from build123d import *

# Parameters (mm, degrees)
SKETCH1_R               = 3
BOSS_EXTRUDE1_DEPTH     = 33
SKETCH2_W               = 1.5
SKETCH2_H               = 4
FILLET2_R               = 0.5
CUT_EXTRUDE2_DEPTH      = 34.271609528
CUT_EXTRUDE2_DEPTH_BACK = 34.271609528
SKETCH3_R               = 1


with BuildPart() as part:
    # Sketch1 → Boss-Extrude1 (new body)
    with BuildSketch(Plane.XY):
        Circle(SKETCH1_R)
    extrude(amount=BOSS_EXTRUDE1_DEPTH)

    # Sketch2 → Cut-Revolve1 (revolve, cut)
    with BuildSketch(Plane(origin=(0, 0, 0), x_dir=(1, 0, 0), z_dir=(0, 1, 0)), mode=Mode.PRIVATE) as cut_revolve1_sk:
        with Locations((2.25, -5)):
            Rectangle(SKETCH2_W, SKETCH2_H)
    revolve(cut_revolve1_sk.sketch.rotate(Axis((0, 0, 0), (0, 0, 1)), 180), axis=Axis((0, 0, 0), (0, 0, 1)), mode=Mode.SUBTRACT)

    # Fillet2
    fillet2_edges = [part.edges().sort_by_distance(p)[0] for p in [
        (-3, 0, 7),
    ]]
    fillet(fillet2_edges, radius=FILLET2_R)

    # Sketch3 → Cut-Extrude2 (cut, two sides: drawn at the far end of the back side and taken through both)
    with BuildSketch(Plane(origin=(0, 0, 0), x_dir=(1, 0, 0), z_dir=(0, 1, 0)).offset(-CUT_EXTRUDE2_DEPTH_BACK)):
        with Locations(Location((0, -30.706648015, 0), (0, 0, 270))):
            Circle(SKETCH3_R)
    extrude(amount=CUT_EXTRUDE2_DEPTH + CUT_EXTRUDE2_DEPTH_BACK, mode=Mode.SUBTRACT)


solid = part.part
Work out the finished part from the listing and answer in its coordinate system (mm). A direction names the side the tool comes from. Give positions to 0.01 mm unless a question says otherwise; leave off trailing zeros. Order: outer loops, then holes, each group sorted by start corner. A loop starts at its lowest first (then second) coordinate and runs counter-clockwise, first axis right, second up. Notation, with made-up numbers: (51.5, 37.25) -> (73.5, 37.25) arc R32 ccw to (73.5, 67.25) -> close; hole circle Ø7 at (18, -30.75). An arc over 180 degrees is marked (long way). One line per item, written item: value.
Item 1: Flat-ended cylindrical pins translate along their axes: P1, Ø3, axis at x = 0, z = 30.71, coming from the -Y side; P2, Ø1.5, axis at y = -1, z = 9, coming from the -X side. Find the tip coordinate at first contact, or state that the pin passes through.
Answer sheet:
P1: y = -3
P2: x = -2.99
Item 2: Find section C-C, the plane z = 3.5. Give the vertices of the cut face in (x, y), plus the area to 3 significant figures.
Answer sheet:
outline: circle Ø3 at (0, 0)
area: 7.07 mm²
Item 3: A tool of negligible diameter and unlimited length cuts with its end or side. For faces 1 (the flat face through (0, 0, 0)), 2 (the flat face through (1.3, 1.3, 3)), from which of +Z, -Z, +X, -X, +Y, -Y can it reach the whole face along a straight path? Write none if from no direction.
Answer sheet:
face 1: -Z, +X, -X, +Y, -Y
face 2: none
Item 4: Find section B-B, the plane y = 0. Give the vertices of the cut face in (x, z).
Answer sheet:
outline: (-3, 0) -> (3, 0) -> (3, 3) -> (1.5, 3) -> (1.5, 7) -> (2.5, 7) arc R0.5 ccw to (3, 7.5) -> (3, 33) -> (-3, 33) -> (-3, 7.5) arc R0.5 ccw to (-2.5, 7) -> (-1.5, 7) -> (-1.5, 3) -> (-3, 3) -> close; hole circle Ø2 at (0, 30.71)
Item 5: Find section A-A, the plane x = 0. Give the vertices of the cut face in (y, z), plus the area to 3 significant figures.
Answer sheet:
outline: (-3, 0) -> (3, 0) -> (3, 3) -> (1.5, 3) -> (1.5, 7) -> (2.5, 7) arc R0.5 ccw to (3, 7.5) -> (3, 29.71) -> (-3, 29.71) -> (-3, 7.5) arc R0.5 ccw to (-2.5, 7) -> (-1.5, 7) -> (-1.5, 3) -> (-3, 3) -> close; (-3, 31.71) -> (3, 31.71) -> (3, 33) -> (-3, 33) -> close
area: 174 mm²
Item 6: Find section D-D, the plane z = 11. Give the vertices of the cut face in (x, y), plus the area to 3 significant figures.
Answer sheet:
outline: circle Ø6 at (0, 0)
area: 28.3 mm²
Item 7: Straight lines are drawn through the part: probe 1 along Z at (x, y) = (0, -2.25); probe 2 along Z at (x, y) = (0, 1); probe 3 along Z at (x, y) = (2.25, 1.25). For each, find the intervals that lie inside material, in ascending order.
Answer sheet:
probe 1: 0 to 3, 7 to 29.71, 31.71 to 33
probe 2: 0 to 29.71, 31.71 to 33
probe 3: 0 to 3, 7.01 to 33
